Verification items for the finished model (mm, model axes). Round coordinates to 2 decimals unless told otherwise and drop trailing zeros. Write each loop counter-clockwise with the first axis right and the second up, starting at its lowest first coordinate (ties: lowest second). Pieces come first, ordered by that corner, then holes. Notation, with made-up numbers: (40.5, 50.5) -> (55.5, 50.5) arc R18 ccw to (55.5, 80.5) -> close; hole circle Ø11 at (5.5, 13.25). An arc over 180 degrees is marked (long way). Answer as a JSON object with one key per item and string values. Group by question number.
(1) Sectioned sample at A-A on x = 20. Record the cut outline in (y, z), and give its area (3 significant figures).
(2) Scan lines: L1, parallel to Y at x = 43.85, z = 42.5 (3 decimals); L2, parallel to Y at x = 5.95, z = 1.2; L3, parallel to Y at x = 5, z = 1. Record each from-to range of solid material in increasing order. Write a range as from..to.
(3) Sectioned sample at B-B on y = 40.9. Record the cut outline in (x, z).
(4) Gauge pin test, flat ends, axial feed: pin 1 Ø0.8 at (y, z) = (4.5, 1) entering from -X; pin 2 Ø2 at (x, z) = (19, 36.5) entering from +Y; pin 3 Ø7 at (x, y) = (5.95, 9.8) entering from -Z; pin 4 Ø21.5 at (x, y) = (27.5, 15) entering from +Z. Record the tip position at first contact, or that the pin passes through.
(5) Sectioned sample at C-C on z = 11.5. Record the cut outline in (x, y), and give its area (3 significant figures).
(6) Sectioned sample at D-D on z = 54. Record the cut outline in (x, y).
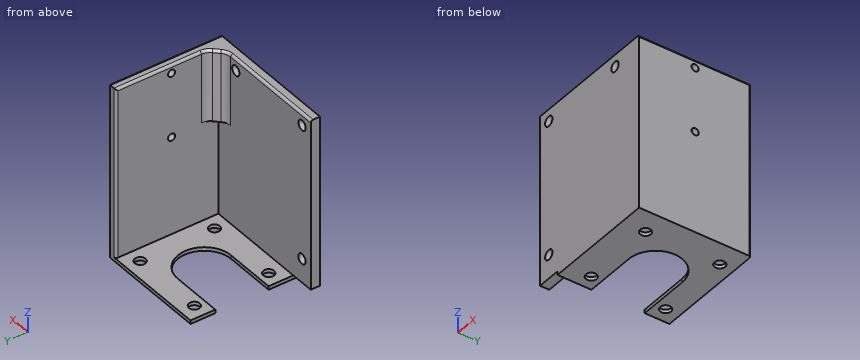
```python
from build123d import *

# Parameters (mm, degrees)
BOSS_EXTRU_1_DEPTH      = 39
ESQUISSE2_R             = 2.25
BOSS_EXTRU_2_DEPTH      = 1.5
ESQUISSE3_W             = 34
ESQUISSE3_H             = 46.85
BOSS_EXTRU_3_DEPTH      = 3.85
ESQUISSE4_R             = 1.5
ENL_V_MAT_EXTRU_1_DEPTH = 6.5
ESQUISSE5_W             = 53
ESQUISSE5_H             = 71.5
BOSS_EXTRU_4_DEPTH      = 3.85
ESQUISSE6_R             = 2.1
ENL_V_MAT_EXTRU_2_DEPTH = 6.5
BOSS_EXTRU_5_DEPTH      = 30
CONG_1_R                = 5
CONG_2_R                = 1


with BuildPart() as part:
    # Esquisse1 → Boss.-Extru.1 (new body)
    with BuildSketch(Plane.XY):
        Polygon((0, 0), (46.85, 0), (46.85, 46.85), (43, 46.85), (43, 3.85), (0, 3.85), align=None)
    extrude(amount=BOSS_EXTRU_1_DEPTH)

    # Esquisse2 → Boss.-Extru.2 (add)
    with BuildSketch(Plane(origin=(0, 0, 0), x_dir=(-1, 0, 0), z_dir=(0, 0, -1))):
        with BuildLine():
            Line((0, 46.85), (-43, 46.85))
            Line((-43, 46.85), (-43, 3.85))
            Line((-43, 3.85), (0, 3.85))
            Line((0, 3.85), (0, 14.2))
            Line((0, 14.2), (-21.5, 14.2))
            ThreePointArc((-21.5, 14.2), (-32.65, 25.35), (-21.5, 36.5))
            Line((-21.5, 36.5), (0, 36.5))
            Line((0, 36.5), (0, 46.85))
        make_face()
        with Locations((-37.05, 9.8)):
            Circle(ESQUISSE2_R, mode=Mode.SUBTRACT)
        with Locations((-5.95, 9.8)):
            Circle(ESQUISSE2_R, mode=Mode.SUBTRACT)
        with Locations((-37.05, 40.9)):
            Circle(ESQUISSE2_R, mode=Mode.SUBTRACT)
        with Locations((-5.95, 40.9)):
            Circle(ESQUISSE2_R, mode=Mode.SUBTRACT)
    extrude(amount=-BOSS_EXTRU_2_DEPTH)

    # Esquisse3 → Boss.-Extru.3 (add)
    with BuildSketch(Plane(origin=(46.85, 0, 0), x_dir=(0, 0, -1), z_dir=(1, 0, 0))):
        with Locations((-56, 23.425)):
            Rectangle(ESQUISSE3_W, ESQUISSE3_H)
    extrude(amount=-BOSS_EXTRU_3_DEPTH)

    # Esquisse4 → Enlèv. mat.-Extru.1 (cut)
    with BuildSketch(Plane(origin=(46.85, 0, 0), x_dir=(0, 0, -1), z_dir=(1, 0, 0))):
        with Locations((-69.5, 23.425)):
            Circle(ESQUISSE4_R)
        with Locations((-42.5, 23.425)):
            Circle(ESQUISSE4_R)
    extrude(amount=-ENL_V_MAT_EXTRU_1_DEPTH, mode=Mode.SUBTRACT)

    # Esquisse5 → Boss.-Extru.4 (add)
    with BuildSketch(Plane(origin=(0, 3.85, 0), x_dir=(1, 0, 0), z_dir=(0, 1, 0))):
        with Locations((16.5, -37.25)):
            Rectangle(ESQUISSE5_W, ESQUISSE5_H)
    extrude(amount=-BOSS_EXTRU_4_DEPTH)

    # Esquisse6 → Enlèv. mat.-Extru.2 (cut)
    with BuildSketch(Plane(origin=(0, 3.85, 0), x_dir=(1, 0, 0), z_dir=(0, 1, 0))):
        with Locations(Location((-5, -68, 0), (0, 0, 180))):
            Circle(ESQUISSE6_R)
        with Locations(Location((33, -68, 0), (0, 0, 180))):
            Circle(ESQUISSE6_R)
        with Locations(Location((-5, -11.5, 0), (0, 0, 180))):
            Circle(ESQUISSE6_R)
    extrude(amount=-ENL_V_MAT_EXTRU_2_DEPTH, mode=Mode.SUBTRACT)

    # Esquisse7 → Boss.-Extru.5 (add)
    with BuildSketch(Plane.XY.offset(73)):
        Polygon((43, 3.85), (43, 8.85), (38, 3.85), align=None)
    extrude(amount=-BOSS_EXTRU_5_DEPTH)

    # Congé1
    cong_1_edges = [part.edges().sort_by_distance(p)[0] for p in [
        (38, 3.85, 58),
        (43, 8.85, 58),
    ]]
    fillet(cong_1_edges, radius=CONG_1_R)

    # Congé2
    cong_2_edges = [part.edges().sort_by_distance(p)[0] for p in [
        (12.964466094, 3.85, 73),
        (43, 46.85, 37.25),
        (46.85, 46.85, 36.5),
        (40.5, 6.35, 73),
        (43, 28.885533906, 73),
        (37.84234935, 4.230602337, 73),
        (42.619397663, 9.00765065, 73),
        (46.85, 23.425, 73),
    ]]
    fillet(cong_2_edges, radius=CONG_2_R)


solid = part.part
```
Computed values:
{
 "1": {"outline": "(0, 0) -> (14.2, 0) -> (14.2, 1.5) -> (3.85, 1.5) -> (3.85, 72) arc R1 ccw to (2.85, 73) -> (0, 73) -> close; (36.5, 0) -> (46.85, 0) -> (46.85, 1.5) -> (36.5, 1.5) -> close", "area": "312 mm2"},
 "2": {"L1": "0..21.925, 24.925..46.839", "L2": "0..7.55, 12.05..14.2, 36.5..38.65, 43.15..46.85", "L3": "0..7.76, 11.84..14.2, 36.5..38.86, 42.94..46.85"},
 "3": {"outline": "(0, 0) -> (3.7, 0) -> (3.7, 1.5) -> (0, 1.5) -> close; (8.2, 0) -> (34.8, 0) -> (34.8, 1.5) -> (8.2, 1.5) -> close; (39.3, 0) -> (46.85, 0) -> (46.85, 72) arc R1 ccw to (45.85, 73) -> (44, 73) arc R1 ccw to (43, 72) -> (43, 1.5) -> (39.3, 1.5) -> close"},
 "4": {"pin 1": "x = 0", "pin 2": "y = 3.85", "pin 3": "z = 0", "pin 4": "z = 1.5"},
 "5": {"outline": "(-10, 0) -> (-7.1, 0) -> (-7.1, 3.85) -> (-10, 3.85) -> close; (-2.9, 0) -> (46.85, 0) -> (46.85, 45.85) arc R1 ccw to (45.85, 46.85) -> (44, 46.85) arc R1 ccw to (43, 45.85) -> (43, 3.85) -> (-2.9, 3.85) -> close", "area": "368 mm2"},
 "6": {"outline": "(-10, 0) -> (46.85, 0) -> (46.85, 45.85) arc R1 ccw to (45.85, 46.85) -> (44, 46.85) arc R1 ccw to (43, 45.85) -> (43, 10.92) arc R5 cw to (41.54, 7.39) -> (39.46, 5.31) arc R5 cw to (35.93, 3.85) -> (-10, 3.85) -> close"}
}
